Autodesk Inventor part; units mm, degrees
ref_plane "YZ Plane" through (0, 0, 0) normal (1, 0, 0) x (0, 1, 0)
ref_plane "XZ Plane" through (0, 0, 0) normal (0, 1, 0) x (-1, 0, 0)
ref_plane "XY Plane" through (0, 0, 0) normal (0, 0, 1) x (1, 0, 0)
sketch "草圖1" plane through (0, 0, 0) normal (0, 1, 0) x (-1, 0, 0)
  line L0 (0, 0) -> (0, -140)
  line L1 (15, -140) -> (15, 0)
  line L2 (6, 0) -> (6, 3)
  line L3 (6, 3) -> (14.1, 3)
  line L4 (14.1, 3) -> (14.1, 0)
  line L5 (15, 0) -> (14.1, 0)
  line L6 (6, 0) -> (0, 0)
  line L7 (6, -140) -> (6, -143)
  line L8 (6, -143) -> (14.1, -143)
  line L9 (14.1, -143) -> (14.1, -140)
  line L10 (0, -140) -> (6, -140)
  line L11 (14.1, -140) -> (15, -140)
  dimension "d1" = 15
  dimension "d2" = 3
  dimension "d3" = 8.1
  dimension "d4" = 6
  dimension "d5" = 3
  dimension "d6" = 140
  dimension "d7" = 6
  dimension "d8" = 8.1
  dimension "d9" = 15
  dimension "d10" = 140
extrude "擠出1" add sketch "草圖1" along normal blind 3
sketch "草圖2" plane through (0, 3, 0) normal (0, 1, 0) x (1, 0, 0)
  line L0 (-11, 1) -> (-8, 1)
  line L1 (-8, 1) -> (-8, 7)
  line L2 (-8, 7) -> (-11, 7)
  line L3 (-11, 7) -> (-11, 1)
  line L4 (0, 0) -> (0, 140)
  line L5 (-6, 0) -> (0, 0)
  line L6 (-11, 133) -> (-8, 133)
  line L7 (-8, 133) -> (-8, 139)
  line L8 (-8, 139) -> (-11, 139)
  line L9 (-11, 139) -> (-11, 133)
  line L10 (0, 140) -> (-6, 140)
  line L11 (-15, 140) -> (-15, 0)
  dimension "d13" = 6
  dimension "d14" = 3
  dimension "d16" = 1
  dimension "d17" = 6
  dimension "d18" = 3
  dimension "d20" = 1
  dimension "d33" = 4
  dimension "d34" = 4
extrude "擠出2" cut sketch "草圖2" against normal up to surface (3 mm away)
sketch "草圖4" plane through (0, 3, 0) normal (0, 1, 0) x (1, 0, 0)
  line L0 (-27, 0) -> (-15, 0)
  line L1 (-15, 0) -> (-15, 140)
  line L2 (-15, 140) -> (-27, 140)
  line L3 (-29, 138) -> (-29, 2)
  line L4 (-15, 140) -> (-15, 0)
  line L5 (0, 140) -> (-6, 140)
  line L6 (-6, 0) -> (0, 0)
  line L7 (-22, 10) -> (-22, 60) construction
  line L8 (-20, 10) -> (-20, 60)
  line L9 (-24, 60) -> (-24, 10)
  arc A0 (-24, 10) -> (-20, 10) centre (-22, 10) ccw
  arc A1 (-20, 60) -> (-24, 60) centre (-22, 60) ccw
  circle A2 centre (-22, 130) radius 2
  arc A3 (-29, 2) -> (-27, 0) centre (-27, 2) ccw
  arc A4 (-27, 140) -> (-29, 138) centre (-27, 138) ccw
  point P0 (-22, 35)
  dimension "d23" = 14
  dimension "d24" = 4
  dimension "d25" = 50
  dimension "d26" = 5
  dimension "d27" = 10
  dimension "d29" = 2
  dimension "d32" = 10
extrude "擠出3" add sketch "草圖4" against normal up to surface (3 mm away)
sketch "草圖6" plane through (0, 3, 0) normal (0, 1, 0) x (1, 0, 0)
  circle A0 centre (-22, 130) radius 2
  arc A1 (-24, 10) -> (-20, 10) centre (-22, 10) ccw
  line L0 (-24, 10) -> (-24, 60)
  arc A2 (-20, 60) -> (-24, 60) centre (-22, 60) ccw
  line L1 (-20, 60) -> (-20, 10)
  line L2 (-8, 7) -> (-8, 1)
  line L3 (-8, 1) -> (-11, 1)
  line L4 (-11, 1) -> (-11, 7)
  line L5 (-11, 7) -> (-8, 7)
  line L6 (-8, 133) -> (-11, 133)
  line L7 (-11, 133) -> (-11, 139)
  line L8 (-11, 139) -> (-8, 139)
  line L9 (-8, 139) -> (-8, 133)
  line L10 (0, 0) -> (0, 140)
  line L11 (0, 140) -> (-6, 140)
  line L12 (-6, 140) -> (-6, 143)
  line L13 (-6, 143) -> (-14.1, 143)
  line L14 (-14.1, 143) -> (-14.1, 140)
  line L15 (-14.1, 140) -> (-27, 140)
  arc A3 (-27, 140) -> (-29, 138) centre (-27, 138) ccw
  line L16 (-29, 138) -> (-29, 2)
  arc A4 (-29, 2) -> (-27, 0) centre (-27, 2) ccw
  line L17 (-27, 0) -> (-14.1, 0)
  line L18 (-14.1, 0) -> (-14.1, -3)
  line L19 (-14.1, -3) -> (-6, -3)
  line L20 (-6, -3) -> (-6, 0)
  line L21 (-6, 0) -> (0, 0)
  line L22 (-6, 140) -> (-6, 143)
  line L23 (-6, 0) -> (-6, 140)
extrude "擠出4" cut sketch "草圖6" against normal blind 3 contours L21 L23 L11 L10
ref_plane "工作平面1" through (-22, 3, -10) normal (1, 0, 0) x (0, 0, -1)
sketch "草圖8" plane through (0, 3, 0) normal (0, 1, 0) x (1, 0, 0)
  line L0 (-14.1, 140) -> (-27, 140)
  line L1 (-14.1, 140) -> (-14.1, 0)
  line L2 (-6, -3) -> (-6, 143)
  line L3 (-6, 143) -> (-14.1, 143)
  line L4 (-14.1, 143) -> (-14.1, 140)
  line L5 (-14.1, 140) -> (-27, 140)
  arc A0 (-27, 140) -> (-29, 138) centre (-27, 138) ccw
  line L6 (-29, 138) -> (-29, 2)
  arc A1 (-29, 2) -> (-27, 0) centre (-27, 2) ccw
  line L7 (-27, 0) -> (-14.1, 0)
  line L8 (-14.1, 0) -> (-14.1, -3)
  line L9 (-14.1, -3) -> (-6, -3)
  circle A2 centre (-22, 130) radius 2
  arc A3 (-24, 10) -> (-20, 10) centre (-22, 10) ccw
  line L10 (-24, 10) -> (-24, 60)
  arc A4 (-20, 60) -> (-24, 60) centre (-22, 60) ccw
  line L11 (-20, 60) -> (-20, 10)
  line L12 (-8, 7) -> (-8, 1)
  line L13 (-8, 1) -> (-11, 1)
  line L14 (-11, 1) -> (-11, 7)
  line L15 (-11, 7) -> (-8, 7)
  line L16 (-8, 133) -> (-11, 133)
  line L17 (-11, 133) -> (-11, 139)
  line L18 (-11, 139) -> (-8, 139)
  line L19 (-8, 139) -> (-8, 133)
  point P0 (0, 0)
extrude "擠出5" cut sketch "草圖8" against normal up to surface (3 mm away) contours L4 L3 L2 L9 L8 L1
equation "\"d10\" = d6"
equation "\"d20\" = d16"
properties part number "chassis_1_2_up"
Could you check a few things on this model? Use its own coordinates, in mm. A direction names the side the tool comes from. Coordinates: 2 decimals unless noted, no trailing zeros. Loops run counter-clockwise (first coordinate to the right, second up) from the corner with the lowest first, then second, coordinate; pieces in that order, holes last. Notation, with made-up numbers: (45, 38) -> (92, 38) arc R8 ccw to (92, 48) -> close; hole circle Ø10 at (27, 45.5). An arc over 180 degrees is marked (long way). Answer in a Markdown table with one row per item.
(1) Imagine slicing it at C-C (y = 1.85). List the corners of the cut face in (x, z) for me.
Results found:
| item | result |
|---|---|
| outline | (-29, -138) arc R2 ccw to (-27, -140) -> (-14.1, -140) -> (-14.1, 0) -> (-27, 0) arc R2 ccw to (-29, -2) -> close; hole circle Ø4 at (-22, -130); hole (-24, -60) arc R2 ccw to (-20, -60) -> (-20, -10) arc R2 ccw to (-24, -10) -> close |
(2) Thinking about a two-plate mould opening in X: for faces 1 (the face through (-21.077, 1.521, -128.226)), 2 (the face through (-29, 2, -71)), 3 (the face through (-20, 2, -140)), 4 (the face through (-24, 2, -35)), which applies, released by +X, released by -X, zero draft, split by the parting line, or undercut?
Results found:
| item | result |
|---|---|
| face 1 | undercut |
| face 2 | released by -X |
| face 3 | zero draft |
| face 4 | undercut |
(3) For faces 5 (the face through (-20, 2, -35)), 6 (the face through (-22, 0, -71)), which set-ups out of +Z, -Z, +X, -X, +Y, -Y let a thin tool reach every point of the face, with its end or its side?
Results found:
| item | result |
|---|---|
| face 5 | +Y, -Y |
| face 6 | +Z, -Z, +X, -X, -Y |
(4) If I drill on probe 1 along Z at (x, y) = (-22, 0.7); probe 2 along Z at (x, y) = (-22.5, 1.9); probe 3 along X at (y, z) = (0.8, -48), over which ranges is the centre line in solid material (lowest first)?
Results found:
| item | result |
|---|---|
| probe 1 | z = -140 to -132, -128 to -62, -8 to 0 |
| probe 2 | z = -140 to -131.94, -128.06 to -61.94, -8.06 to 0 |
| probe 3 | x = -29 to -24, -20 to -14.1 |
(5) Imagine slicing it at A-A (x = -22). List the corners of the cut face in (y, z) for me.
Results found:
| item | result |
|---|---|
| outline | (0, -140) -> (3, -140) -> (3, -132) -> (0, -132) -> close; (0, -128) -> (3, -128) -> (3, -62) -> (0, -62) -> close; (0, -8) -> (3, -8) -> (3, 0) -> (0, 0) -> close |
(6) Imagine slicing it at B-B (z = -130). List the corners of the cut face in (x, y) for me.
Results found:
| item | result |
|---|---|
| outline | (-29, 0) -> (-24, 0) -> (-24, 3) -> (-29, 3) -> close; (-20, 0) -> (-14.1, 0) -> (-14.1, 3) -> (-20, 3) -> close |
